Part model, mm, in its own coordinate system. Face numbers are marked on the shaded views. A direction names the side the tool comes from. Coordinates: 2 decimals unless noted, no trailing zeros. Loops run counter-clockwise (first coordinate to the right, second up) from the corner with the lowest first, then second, coordinate; pieces in that order, holes last. Notation, with made-up numbers: (-6.75, -14) - (49.25, -14) arc R15 cw to (49.25, -5) - close; hole circle Ø8 at (82, 68.5). An arc over 180 degrees is marked (long way). Use a Markdown table: item, result. Add a question column.
1. Band-saw the part on C-C, the plane z = -18. Give the cut face in (x, y).
2. Wall check: probe 1 along Y at (x, z) = (-2, -11); probe 2 along X at (y, z) = (33, -25.5); probe 3 along X at (y, z) = (46, -36). Give the ranges that are in metal, low to high. Write a range as [from, to].
3. Pull direction Y, two halves, no side cores. Call the marked faces 1, 2, 3 and 4: pulls with the +Y half, pulls with the -Y half, needs draft (parallel to the pull), parting line crosses it, or undercut.
4. Band-saw the part on A-A, the plane z = -25. Give the cut face in (x, y).
5. Band-saw the part on D-D, the plane x = 11.5. Give the cut face in (y, z), plus the area to 3 significant figures.
6. 3-axis set-ups, long thin cutter, end or side, ignore diameter. For the marked faces 5, 6 and 7: which of +Z, -Z, +X, -X, +Y, -Y reach the whole face in a straight line?
7. Drop flat-ended pins along their axis: pin 1 (3 mm diameter, centred on x = 15.5, y = 29, fed in from -Z); pin 2 (0.6 mm diameter, centred on x = 1.5, z = -25.5, fed in from -Y). Give the stop position or say it passes through.
8. Band-saw the part on B-B, the plane y = 32.5. Give the cut face in (x, z), plus the area to 3 significant figures.
from build123d import *

# Parameters (mm, degrees)
F0_R      = 1.75
F1_DEPTH  = 15
F2_W      = 42
F2_H      = 30
F2_H_2    = 45
F3_DEPTH  = 10
F4_W      = 42
F4_H      = 40
F4_R      = 2.25
F5_DEPTH  = 10
F6_R      = 2
F7_DEPTH  = 25
F8_R      = 2
F9_DEPTH  = 12
F11_DEPTH = 8.5
F12_R     = 6
F13_DEPTH = 9
F14_R     = 8
F15_DEPTH = 3.4
F16_W     = 16
F16_H     = 8.6135048579
F17_DEPTH = 12
F18_R     = 1.75
F19_DEPTH = 55
F21_DEPTH = 5
F22_W     = 1.8
F22_H     = 3.5010978645
F23_DEPTH = 25


with BuildPart() as f1:
    # F0 (on Front) → F1 (new body)
    with BuildSketch(Plane.XZ):
        with BuildLine():
            Line((-21, -21), (21, -21))
            Line((21, -21), (21, -10))
            Line((21, -10), (4.582575695, -10))
            ThreePointArc((4.582575695, -10), (0, -11), (-4.582575695, -10))
            Line((-4.582575695, -10), (-21, -10))
            Line((-21, -10), (-21, -21))
        make_face()
        with Locations((-15.5, -15.5)):
            Circle(F0_R, mode=Mode.SUBTRACT)
        with Locations((15.5, -15.5)):
            Circle(F0_R, mode=Mode.SUBTRACT)
    extrude(amount=-F1_DEPTH)

    # F2 (on face) → F3 (join)
    with BuildSketch(Plane(origin=(0, 0, -21), x_dir=(1, 0, 0), z_dir=(0, 0, -1))):
        with Locations((0, -30)):
            Rectangle(F2_W, F2_H)
        with Locations((0, -22.5)):
            Rectangle(F2_W, F2_H_2)
    extrude(amount=F3_DEPTH)

    # F4 (on face) → F5 (join)
    with BuildSketch(Plane(origin=(0, 45, 0), x_dir=(-1, 0, 0), z_dir=(0, 1, 0))):
        with Locations((0, -20)):
            Rectangle(F4_W, F4_H)
        with Locations((-11.5, -33.9412614703)):
            Circle(F4_R, mode=Mode.SUBTRACT)
        with Locations((11.5, -33.9412614703)):
            Circle(F4_R, mode=Mode.SUBTRACT)
        with Locations((-11.5, -10.9412614703)):
            Circle(F4_R, mode=Mode.SUBTRACT)
        with Locations((11.5, -10.9412614703)):
            Circle(F4_R, mode=Mode.SUBTRACT)
    extrude(amount=F5_DEPTH)

    # F6 (on face) → F7 (cut)
    with BuildSketch(Plane.XY.offset(-10)):
        with Locations((-5, 5.3)):
            Circle(F6_R)
    extrude(amount=-F7_DEPTH, mode=Mode.SUBTRACT)

    # F8 (on face) → F9 (cut)
    with BuildSketch(Plane(origin=(0, 0, -31), x_dir=(1, 0, 0), z_dir=(0, 0, -1))):
        with BuildLine():
            ThreePointArc((-10.9924953066, 0), (-7.8337287756, -12.781308791), (3, -5.3))
            ThreePointArc((3, -5.3), (2.481308791, -2.4662712244), (0.9924953066, 0))
            Line((0.9924953066, 0), (-10.9924953066, 0))
        make_face()
        with Locations((-5, -5.3)):
            Circle(F8_R, mode=Mode.SUBTRACT)
    extrude(amount=-F9_DEPTH, mode=Mode.SUBTRACT)

    # F10 (on face) → F11 (join)
    with BuildSketch(Plane(origin=(0, 0, -31), x_dir=(1, 0, 0), z_dir=(0, 0, -1))):
        with BuildLine():
            ThreePointArc((-10.9924953066, 0), (-7.8337287756, -12.781308791), (3, -5.3))
            ThreePointArc((3, -5.3), (2.481308791, -2.4662712244), (0.9924953066, 0))
            ThreePointArc((0.9924953066, 0), (-5, 2.7), (-10.9924953066, 0))
        make_face()
    extrude(amount=-F11_DEPTH)

    # F12 (on face) → F13 (cut)
    with BuildSketch(Plane(origin=(0, 0, -31), x_dir=(1, 0, 0), z_dir=(0, 0, -1))):
        with Locations((-5, -5.3)):
            Circle(F12_R)
    extrude(amount=-F13_DEPTH, mode=Mode.SUBTRACT)

    # F14 (on face) → F15 (cut)
    with BuildSketch(Plane(origin=(0, 0, -31), x_dir=(1, 0, 0), z_dir=(0, 0, -1))):
        with Locations((-5, -5.3)):
            Circle(F14_R)
    extrude(amount=-F15_DEPTH, mode=Mode.SUBTRACT)

    # F16 (on face) → F17 (cut)
    with BuildSketch(Plane(origin=(0, 0, -31), x_dir=(1, 0, 0), z_dir=(0, 0, -1))):
        with Locations((-5, -0.993247571)):
            Rectangle(F16_W, F16_H)
    extrude(amount=-F17_DEPTH, mode=Mode.SUBTRACT)

    # F18 (on face) → F19 (cut)
    with BuildSketch(Plane.XZ):
        with Locations((-15.9438401461, -25)):
            Circle(F18_R)
        with Locations((7.0561598539, -25)):
            Circle(F18_R)
    extrude(amount=-F19_DEPTH, mode=Mode.SUBTRACT)

    # F20 (on face) → F21 (cut)
    with BuildSketch(Plane.XZ.offset(-45)):
        Polygon((-10.8610754958, -14.9911720222), (-7.673212327, -12.4128918945), (-8.3121368311, -8.3629813427), (-12.1389245042, -6.8913509185), (-15.326787673, -9.4696310461), (-14.6878631689, -13.519541598), align=None)
        Polygon((9.9157388399, -14.7228109644), (13.9827873475, -14.2040466283), (15.5670485076, -10.4224971341), (13.0842611601, -7.1597119762), (9.0172126525, -7.6784763124), (7.4329514924, -11.4600258065), align=None)
    extrude(amount=-F21_DEPTH, mode=Mode.SUBTRACT)

    # F22 (on face) → F23 (cut)
    with BuildSketch(Plane.XY.offset(-10)):
        with Locations((-4.9740429662, 1.7505489322)):
            Rectangle(F22_W, F22_H)
    extrude(amount=-F23_DEPTH, mode=Mode.SUBTRACT)


solid = f1.part
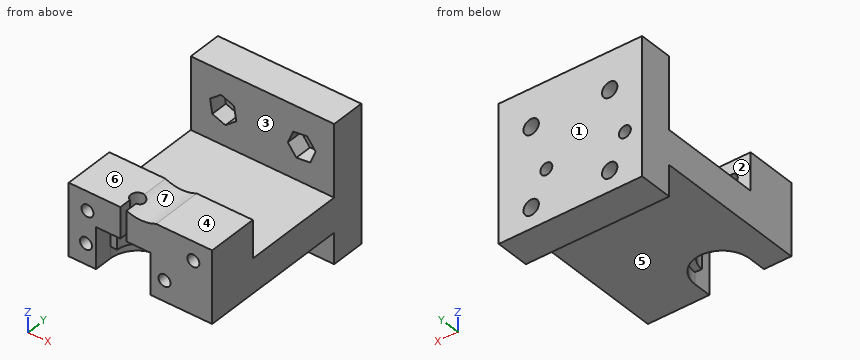
Geometry check:
| question | item | result |
|---|---|---|
| 1 | outline | (-21, 0) - (-5.87, 0) - (-5.87, 3.5) arc R2 cw (long way) to (-4.13, 3.5) - (-4.07, 3.5) - (-4.07, 0) - (21, 0) - (21, 15) - (-21, 15) - close; (-21, 45) - (21, 45) - (21, 55) - (-21, 55) - close |
| 2 | probe 1 | y = [0, 15], [45, 55] |
| 2 | probe 2 | x = [-21, -17.62], [-14.27, 5.38], [8.73, 21] |
| 2 | probe 3 | x = [-21, -12.41], [-10.59, 10.59], [12.41, 21] |
| 3 | face 1 | pulls with the +Y half |
| 3 | face 2 | undercut |
| 3 | face 3 | undercut |
| 3 | face 4 | needs draft |
| 4 | outline | (-21, 0) - (-17.69, 0) - (-17.69, 55) - (-21, 55) - close; (-14.19, 0) - (-13, 0) - (-13, 5.3) - (-11, 5.3) arc R6 cw to (1, 5.3) - (3, 5.3) - (3, 0) - (5.31, 0) - (5.31, 55) - (-14.19, 55) - close; (8.81, 0) - (21, 0) - (21, 55) - (8.81, 55) - close |
| 5 | outline | (0, -31) - (45, -31) - (45, -31.69) - (55, -31.69) - (55, -13.19) - (50, -13.19) - (50, -14.52) - (45, -14.52) - (45, -21) - (15, -21) - (15, -10) - (0, -10) - close; (45, -40) - (55, -40) - (55, -36.19) - (45, -36.19) - close; (45, -7.36) - (50, -7.36) - (50, -8.69) - (55, -8.69) - (55, 0) - (45, 0) - close |
| 5 | area | 912 mm^2 |
| 6 | face 5 | -Z, +X, -X, -Y |
| 6 | face 6 | +Z, +X, -X, -Y |
| 6 | face 7 | +Z, -Y |
| 7 | pin 1 | stops at z = -31 |
| 7 | pin 2 | stops at y = 5.3 |
| 8 | outline | (-21, -31) - (21, -31) - (21, -21) - (-21, -21) - close; hole circle Ø3.5 at (-15.94, -25); hole circle Ø3.5 at (7.06, -25) |
| 8 | area | 401 mm^2 |
